Here's how the part is built. I have some questions about the finished solid (model axes, mm). A direction names the side the tool comes from. Round coordinates to 2 decimals unless told otherwise and drop trailing zeros. Loops run counter-clockwise (first coordinate to the right, second up) from the corner with the lowest first, then second, coordinate; pieces in that order, holes last. Notation, with made-up numbers: M 47.5,5 L 103.5,5 A24 ccw 103.5,26 Z; hole C 29.25,25 d6. An arc over 180 degrees is marked long. Answer as a JSON object with one key per item and string values.
from build123d import *

# Parameters (mm, degrees)
SKETCH_1_R          = 9
SKETCH_1_R_2        = 7.5
EXTRUDE_1_DEPTH     = 6
EXTRUDE_START       = -1
EXTRUDE_2_DEPTH     = 1
EXTRUDE_3_DEPTH     = 3
EXTRUDE_START_2     = -3
SKETCH_5_R          = 7.5
EXTRUDE_4_DEPTH     = 3
SKETCH_6_R          = 1.6
CUT_EXTRUDE_1_DEPTH = 3
CHAMFER_1_SIZE      = 1
SKETCH_14_R         = 1.1
CUT_EXTRUDE_4_DEPTH = 1.5


with BuildPart() as part:
    # 草图1 → 凸台-拉伸1 (new body)
    with BuildSketch(Plane(origin=(0, 0, 0), x_dir=(1, 0, 0), z_dir=(0, 1, 0))):
        with Locations(Location((0, 0, 0), (0, 0, 270))):
            Circle(SKETCH_1_R)
        with Locations(Location((0, 0, 0), (0, 0, 270))):
            Circle(SKETCH_1_R_2, mode=Mode.SUBTRACT)
    extrude(amount=EXTRUDE_1_DEPTH)

    # 草图2 → 凸台-拉伸2 (add)
    with BuildSketch(Plane(origin=(0, 6, 0), x_dir=(1, 0, 0), z_dir=(0, 1, 0)).offset(EXTRUDE_START)):
        with BuildLine():
            Line((-19.923893962, 1.743114855), (-8.965752283, 0.784401685))
            ThreePointArc((-8.965752283, 0.784401685), (0.392574486, 8.991433994), (9, 0))
            ThreePointArc((9, 0), (0.392574486, -8.991433994), (-8.965752283, -0.784401685))
            Line((-8.965752283, -0.784401685), (-19.923893962, -1.743114855))
            ThreePointArc((-19.923893962, -1.743114855), (0.872387747, -19.980964432), (20, 0))
            ThreePointArc((20, 0), (0.872387747, 19.980964432), (-19.923893962, 1.743114855))
        make_face()
    extrude(amount=EXTRUDE_2_DEPTH)

    # 草图4 → 凸台-拉伸3 (add)
    with BuildSketch(Plane.XZ):
        with BuildLine():
            Line((0.856553191, 6.326082651), (0.856553191, 7.450927233))
            ThreePointArc((0.856553191, 7.450927233), (-0.043739259, 7.499872457), (-0.943399591, 7.440429908))
            Line((-0.943399591, 7.440429908), (-0.943399591, 6.312339741))
            Line((-0.943399591, 6.312339741), (-0.943399591, 5.418486616))
            ThreePointArc((-0.943399591, 5.418486616), (-0.044016518, 5.499823865), (0.856553191, 5.432892106))
            Line((0.856553191, 5.432892106), (0.856553191, 6.326082651))
        make_face()
        with BuildLine():
            Line((6.312339741, 0.943399591), (5.418486616, 0.943399591))
            ThreePointArc((5.418486616, 0.943399591), (5.499823865, 0.044016518), (5.432892106, -0.856553191))
            Line((5.432892106, -0.856553191), (6.326082651, -0.856553191))
            Line((6.326082651, -0.856553191), (7.450927233, -0.856553191))
            ThreePointArc((7.450927233, -0.856553191), (7.499872457, 0.043739259), (7.440429908, 0.943399591))
            Line((7.440429908, 0.943399591), (6.312339741, 0.943399591))
        make_face()
        with BuildLine():
            Line((0.943399591, -6.312339741), (0.943399591, -5.418486616))
            ThreePointArc((0.943399591, -5.418486616), (0.044016518, -5.499823865), (-0.856553191, -5.432892106))
            Line((-0.856553191, -5.432892106), (-0.856553191, -6.326082651))
            Line((-0.856553191, -6.326082651), (-0.856553191, -7.450927233))
            ThreePointArc((-0.856553191, -7.450927233), (0.043739259, -7.499872457), (0.943399591, -7.440429908))
            Line((0.943399591, -7.440429908), (0.943399591, -6.312339741))
        make_face()
        with BuildLine():
            Line((-6.312339741, -0.943399591), (-5.418486616, -0.943399591))
            ThreePointArc((-5.418486616, -0.943399591), (-5.499823865, -0.044016518), (-5.432892106, 0.856553191))
            Line((-5.432892106, 0.856553191), (-6.326082651, 0.856553191))
            Line((-6.326082651, 0.856553191), (-7.450927233, 0.856553191))
            ThreePointArc((-7.450927233, 0.856553191), (-7.499872457, -0.043739259), (-7.440429908, -0.943399591))
            Line((-7.440429908, -0.943399591), (-6.312339741, -0.943399591))
        make_face()
    extrude(amount=-EXTRUDE_3_DEPTH)

    # 草图5 → 凸台-拉伸4 (add)
    with BuildSketch(Plane(origin=(0, 6, 0), x_dir=(1, 0, 0), z_dir=(0, 1, 0)).offset(EXTRUDE_START_2)):
        Circle(SKETCH_5_R)
    extrude(amount=EXTRUDE_4_DEPTH)

    # 草图6 → 切除-拉伸1 (cut)
    with BuildSketch(Plane(origin=(0, 6, 0), x_dir=(1, 0, 0), z_dir=(0, 1, 0))):
        with Locations(Location((0, 0, 0), (0, 0, 270))):
            Circle(SKETCH_6_R)
    extrude(amount=-CUT_EXTRUDE_1_DEPTH, mode=Mode.SUBTRACT)

    # 倒角1
    chamfer_1_edges = [part.edges().sort_by_distance(p)[0] for p in [
        (0, 0, -9),
    ]]
    chamfer(chamfer_1_edges, length=CHAMFER_1_SIZE)

    # 草图14 → 切除-拉伸4 (cut)
    with BuildSketch(Plane(origin=(0, 6, 0), x_dir=(1, 0, 0), z_dir=(0, 1, 0))):
        with Locations(Location((0, 4.5, 0), (0, 0, 270))):
            Circle(SKETCH_14_R)
        with Locations(Location((4.5, 0, 0), (0, 0, 270))):
            Circle(SKETCH_14_R)
        with Locations(Location((0, -4.5, 0), (0, 0, 270))):
            Circle(SKETCH_14_R)
        with Locations(Location((-4.5, 0, 0), (0, 0, 270))):
            Circle(SKETCH_14_R)
    extrude(amount=-CUT_EXTRUDE_4_DEPTH, mode=Mode.SUBTRACT)


solid = part.part
Item 1: I want a section at D-D on x = 15.5. List the corners of the cut face in (y, z) for me, plus the area to 3 significant figures.
Solution:
{"outline": "M 5,-12.64 L 6,-12.64 L 6,12.64 L 5,12.64 Z", "area": "25.3 mm2"}
Item 2: I want a section at A-A on y = 2.2. List the corners of the cut face in (x, z) for me.
Solution:
{"outline": "C 0,0 d18; hole M -7.45,0.86 L -5.43,0.86 A5.5 ccw -5.42,-0.94 L -7.44,-0.94 A7.5 ccw -0.86,-7.45 L -0.86,-5.43 A5.5 ccw 0.94,-5.42 L 0.94,-7.44 A7.5 ccw 7.45,-0.86 L 5.43,-0.86 A5.5 ccw 5.42,0.94 L 7.44,0.94 A7.5 ccw 0.86,7.45 L 0.86,5.43 A5.5 ccw -0.94,5.42 L -0.94,7.44 A7.5 ccw Z"}
Item 3: I want a section at B-B on x = 0. List the corners of the cut face in (y, z) for me.
Solution:
{"outline": "M 0,-8 L 1,-9 L 5,-9 L 5,-20 L 6,-20 L 6,-5.6 L 4.5,-5.6 L 4.5,-3.4 L 6,-3.4 L 6,-1.6 L 3,-1.6 L 3,-5.5 L 0,-5.5 Z; M 0,5.5 L 3,5.5 L 3,1.6 L 6,1.6 L 6,3.4 L 4.5,3.4 L 4.5,5.6 L 6,5.6 L 6,20 L 5,20 L 5,9 L 1,9 L 0,8 Z"}
Item 4: I want a section at C-C on z = -16. List the corners of the cut face in (x, y) for me, plus the area to 3 significant figures.
Solution:
{"outline": "M -12,5 L 12,5 L 12,6 L -12,6 Z", "area": "24.0 mm2"}
Item 5: For P1, Ø1, axis at x = -7, y = 2, coming from the +Z side; P2, Ø1, axis at y = 1, z = 6.5, coming from the +X side; P3, Ø1, axis at y = 2, z = -5.5, coming from the -X side, each with a flat end and sliding along its axis, tell me the tip position at first contact or that it passes through.
Solution:
{"P1": "stops at z = 6.22", "P2": "stops at x = 6.71", "P3": "stops at x = -7.48"}
Item 6: For faces 3 (the face through (-0.97, 4.52, -1.27)), 4 (the face through (0, 4.5, 4)), 5 (the face through (-5.5, 1.5, -0.1)), which set-ups out of +Z, -Z, +X, -X, +Y, -Y let a thin tool reach every point of the face, with its end or its side?
Solution:
{"face 3": "+Y, -Y", "face 4": "+Y", "face 5": "-Y"}
Item 7: If I drill on L1, parallel to X at y = 5.35, z = 0; L2, parallel to X at y = 0.55, z = 6; L3, parallel to Y at x = 10, z = -1.5, over which ranges is the centre line in solid material (lowest first)? Write a range as from..to.
Solution:
{"L1": "x = -9..-5.6, -3.4..-1.6, 1.6..3.4, 5.6..20", "L2": "x = -6.09..-4.5, -0.94..0.86, 4.5..6.09", "L3": "y = 5..6"}
Item 8: We'd pull the mould along X, two halves only. Please class faces 1 (the face through (0, 0, 6)), 2 (the face through (-5.383, 1.479, 5.222)): +X half, -X half, draft (parallel to the pull), parting line (faces both ways), or undercut.
Solution:
{"face 1": "draft", "face 2": "undercut"}
